```python
from build123d import *

# Parameters (mm, degrees)
SKETCH1_R           = 1.75
BOSS_EXTRUDE1_DEPTH = 10
BOSS_EXTRUDE2_DEPTH = 10


with BuildPart() as part:
    # Sketch1 → Boss-Extrude1 (new body)
    with BuildSketch(Plane.XY):
        Polygon((-2.419560872, 1), (11, 1), (11, 8), (11, 63), (-9, 63), (-9, 56), (5, 56), (5, 8), (-9, 8), (-9, 1), align=None)
        with Locations((-5.5, 59.5)):
            Circle(SKETCH1_R, mode=Mode.SUBTRACT)
        with Locations((8, 54)):
            Circle(SKETCH1_R, mode=Mode.SUBTRACT)
        with Locations((-5.5, 4.5)):
            Circle(SKETCH1_R, mode=Mode.SUBTRACT)
        with Locations((8, 10)):
            Circle(SKETCH1_R, mode=Mode.SUBTRACT)
        with Locations((8, 32)):
            Circle(SKETCH1_R, mode=Mode.SUBTRACT)
    extrude(amount=BOSS_EXTRUDE1_DEPTH)

    # Sketch2 → Boss-Extrude2 (add)
    with BuildSketch(Plane.XY.offset(10)):
        Polygon((5, 42), (5, 48), (-25, 48), (-25, 63), (-35, 63), (-35, 16), (5, 16), (5, 22), (-25, 22), (-25, 42), align=None)
    extrude(amount=-BOSS_EXTRUDE2_DEPTH)


solid = part.part
```
Part model, mm, in its own coordinate system. A direction names the side the tool comes from. Round coordinates to 2 decimals unless told otherwise and drop trailing zeros. Write each loop counter-clockwise with the first axis right and the second up, starting at its lowest first coordinate (ties: lowest second). Pieces come first, ordered by that corner, then holes.
Item 1: Cut at A-A, the plane y = 32. Give the cut face in (x, z).
Results:
outline: (-35, 0) - (-25, 0) - (-25, 10) - (-35, 10) - close; (5, 0) - (6.25, 0) - (6.25, 10) - (5, 10) - close; (9.75, 0) - (11, 0) - (11, 10) - (9.75, 10) - close
Item 2: Probe L1, parallel to Y at x = 8, z = 3.75; L2, parallel to Y at x = -5.5, z = 3.25; L3, parallel to Y at x = -14, z = 9. List the from-to ranges inside material, lowest first.
Results:
L1: y = 1 to 8.25, 11.75 to 30.25, 33.75 to 52.25, 55.75 to 63
L2: y = 1 to 2.75, 6.25 to 8, 16 to 22, 42 to 48, 56 to 57.75, 61.25 to 63
L3: y = 16 to 22, 42 to 48
Item 3: Drop a flat-ended pin along its axis: pin 1 Ø2 at (y, z) = (4.5, 6) entering from -X. Give the stop position or say it passes through.
Results:
pin 1: stops at x = -9
Item 4: Which spindle directions (+Z, -Z, +X, -X, +Y, -Y) get a long thin tool onto all of the face, cutting with end or side? Do faces 1 (the flat face through (-25, 55, 5)), 2 (the flat face through (5, 12, 5)), 3 (the flat face through (-10, 22, 5)). Say none if no direction does.
Results:
face 1: +Z, -Z, +Y
face 2: +Z, -Z, -X
face 3: +Z, -Z
Item 5: Two-plate mould, pull along X, no slides. Class faces 4 (the cylindrical face through (8.9, 11.5, 4.9)), 5 (the flat face through (-9, 5, 5)), 6 (the flat face through (-15, 16, 5)): +X half, -X half, draft (parallel to the pull), parting line (faces both ways), or undercut.
Results:
face 4: undercut
face 5: -X half
face 6: draft
Item 6: Cut at C-C, the plane z = 4. Give the cut face in (x, y), plus the area to 3 significant figures.
Results:
outline: (-35, 16) - (5, 16) - (5, 8) - (-9, 8) - (-9, 1) - (11, 1) - (11, 63) - (-9, 63) - (-9, 56) - (5, 56) - (5, 48) - (-25, 48) - (-25, 63) - (-35, 63) - close; hole (-25, 22) - (5, 22) - (5, 42) - (-25, 42) - close; hole circle Ø3.5 at (-5.5, 4.5); hole circle Ø3.5 at (-5.5, 59.5); hole circle Ø3.5 at (8, 10); hole circle Ø3.5 at (8, 32); hole circle Ø3.5 at (8, 54)
area: 1,350 mm2
Item 7: Cut at B-B, the plane x = -22. Give the cut face in (y, z), plus the area to 3 significant figures.
Results:
outline: (16, 0) - (22, 0) - (22, 10) - (16, 10) - close; (42, 0) - (48, 0) - (48, 10) - (42, 10) - close
area: 120 mm2
Item 8: Cut at D-D, the plane y = 10. Give the cut face in (x, z).
Results:
outline: (5, 0) - (6.25, 0) - (6.25, 10) - (5, 10) - close; (9.75, 0) - (11, 0) - (11, 10) - (9.75, 10) - close
